Work out the finished part from the listing and answer in its coordinate system (mm). Face numbers are marked on the shaded views. A direction names the side the tool comes from. Give positions to 0.01 mm unless a question says otherwise; leave off trailing zeros. Loops run counter-clockwise (first coordinate to the right, second up) from the corner with the lowest first, then second, coordinate; pieces in that order, holes last. Notation, with made-up numbers: M -32,32 L 24,32 A25 ccw 24,60 Z; hole C 18,-15.5 d8. An arc over 180 degrees is marked long. Write item = value, one per line. Start each with the question number.
1. Consider L1, parallel to X at y = 19, z = 1.5; L2, parallel to X at y = 40.5, z = -5.5; L3, parallel to X at y = 40, z = -1.75. Determine where each line is inside the solid, lowest interval first. Write a range as [from, to].
2. For the marked faces 1, 2 and 3, determine the directions among +Z, -Z, +X, -X, +Y, -Y from which every point of the face is accessible in a straight line to the end or side of a thin tool.
3. Flat-ended cylindrical pins translate along their axes: pin 1 Ø1.8 at (x, y) = (761.67, 40.98) entering from -Z; pin 2 Ø4.5 at (y, z) = (38.5, -6) entering from +X; pin 3 Ø4 at (x, z) = (755, -5.5) entering from -Y; pin 4 Ø6 at (x, z) = (739, 0) entering from +Y. Find the tip coordinate at first contact, or state that the pin passes through.
4. Section C-C on y = 17 is taken. Determine the outline of the cut face in (x, z).
5. Section D-D on x = 738 is taken. Determine the outline of the cut face in (y, z), plus the area to 3 significant figures.
6. The mould has two halves that part along Y. Classify the marked faces 4, 5 and 6: released by +Y, released by -Y, zero draft, split by the parting line, or undercut.
7. Section A-A on x = 750 is taken. Determine the outline of the cut face in (y, z).
8. Section B-B on z = -5 is taken. Determine the outline of the cut face in (x, y).
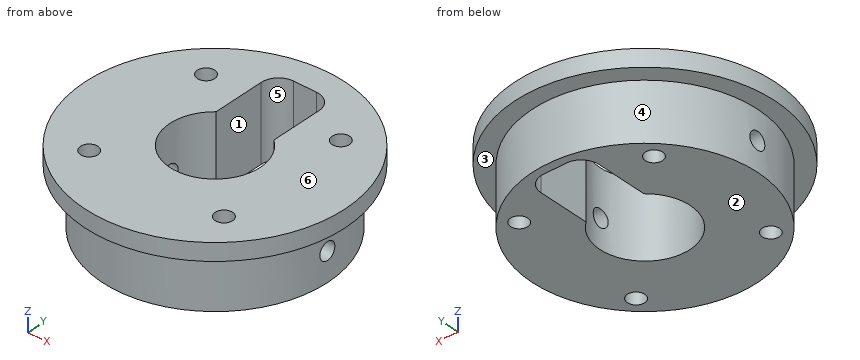
```python
from build123d import *

# Parameters (mm, degrees)
SKETCH1_R               = 22.5
BOSS_EXTRUDE1_DEPTH     = 3
SKETCH2_R               = 19.5
BOSS_EXTRUDE2_DEPTH     = 10
SKETCH3_R               = 1.5
CUT_EXTRUDE1_DEPTH      = 13
CUT_EXTRUDE2_DEPTH      = 60.505474974
CUT_EXTRUDE2_DEPTH_BACK = 60.505474974
SKETCH4_R               = 1.5


with BuildPart() as part:
    # Sketch1 → Boss-Extrude1 (new body)
    with BuildSketch(Plane.XY):
        with Locations((750, 29.313623227)):
            Circle(SKETCH1_R)
    extrude(amount=BOSS_EXTRUDE1_DEPTH)

    # Sketch2 → Boss-Extrude2 (add)
    with BuildSketch(Plane(origin=(0, 0, 0), x_dir=(-1, 0, 0), z_dir=(0, 0, -1))):
        with Locations((-750, 29.313623227)):
            Circle(SKETCH2_R)
    extrude(amount=BOSS_EXTRUDE2_DEPTH)

    # Sketch3 → Cut-Extrude1 (cut)
    with BuildSketch(Plane.XY.offset(3)):
        with Locations((761.66726189, 17.646361337)):
            Circle(SKETCH3_R)
        with Locations((738.33273811, 17.646361337)):
            Circle(SKETCH3_R)
        with Locations((738.33273811, 40.980885116)):
            Circle(SKETCH3_R)
        with Locations((761.66726189, 40.980885116)):
            Circle(SKETCH3_R)
        with BuildLine():
            Line((748, 47.313623227), (752, 47.313623227))
            ThreePointArc((752, 47.313623227), (754.121320344, 46.43494357), (755, 44.313623227))
            Line((755, 44.313623227), (755, 35.313623227))
            ThreePointArc((755, 35.313623227), (750, 21.503373551), (745, 35.313623227))
            Line((745, 35.313623227), (745, 44.313623227))
            ThreePointArc((745, 44.313623227), (745.878679656, 46.43494357), (748, 47.313623227))
        make_face()
    extrude(amount=-CUT_EXTRUDE1_DEPTH, mode=Mode.SUBTRACT)

    # Sketch4 → Cut-Extrude2 (cut, two sides: drawn at the far end of the back side and taken through both)
    with BuildSketch(Plane(origin=(745, 0, 0), x_dir=(0, 0, -1), z_dir=(1, 0, 0)).offset(-CUT_EXTRUDE2_DEPTH_BACK)):
        with Locations((5, 29.313623227)):
            Circle(SKETCH4_R)
    extrude(amount=CUT_EXTRUDE2_DEPTH + CUT_EXTRUDE2_DEPTH_BACK, mode=Mode.SUBTRACT)


solid = part.part
```
Verdict:
q1.L1 = [730, 737.69], [738.98, 761.02], [762.31, 770]
q1.L2 = [734.03, 736.91], [739.75, 745], [755, 760.25], [763.09, 765.97]
q1.L3 = [733.69, 737.2], [739.47, 745], [755, 760.53], [762.8, 766.31]
q2.face_1 = +Z, -Z
q2.face_2 = -Z, +X, -X, +Y, -Y
q2.face_3 = -Z
q3.pin_1 = through
q3.pin_2 = 768.22
q3.pin_3 = 10.05
q3.pin_4 = 50.34
q4.outline = M 731.17,0 L 734.88,0 L 734.88,-10 L 736.98,-10 L 736.98,3 L 731.17,3 Z; M 739.69,-10 L 760.31,-10 L 760.31,3 L 739.69,3 Z; M 763.02,-10 L 765.12,-10 L 765.12,0 L 768.83,0 L 768.83,3 L 763.02,3 Z
q5.outline = M 10.28,0 L 13.94,0 L 13.94,-10 L 16.18,-10 L 16.18,3 L 10.28,3 Z; M 19.11,-10 L 39.52,-10 L 39.52,3 L 19.11,3 Z; M 42.44,-10 L 44.68,-10 L 44.68,0 L 48.35,0 L 48.35,3 L 42.44,3 Z; hole C 29.31,-5 d3
q5.area = 338 mm2
q6.face_4 = split by the parting line
q6.face_5 = undercut
q6.face_6 = zero draft
q7.outline = M 6.81,0 L 9.81,0 L 9.81,-10 L 21.5,-10 L 21.5,3 L 6.81,3 Z; M 47.31,-10 L 48.81,-10 L 48.81,0 L 51.81,0 L 51.81,3 L 47.31,3 Z
q8.outline = M 730.56,27.81 A19.5 ccw 769.44,27.81 L 757.66,27.81 A7.81 cw 742.34,27.81 Z; M 730.56,30.81 L 742.34,30.81 A7.81 cw 745,35.31 L 745,44.31 A3 cw 748,47.31 L 752,47.31 A3 cw 755,44.31 L 755,35.31 A7.81 cw 757.66,30.81 L 769.44,30.81 A19.5 ccw Z; hole C 738.33,17.65 d3; hole C 738.33,40.98 d3; hole C 761.67,17.65 d3; hole C 761.67,40.98 d3
